The drawing under review shows one solid part. Ordinate dimensions are in mm from its lowest x, y, z. Coordinates: 2 decimals unless noted, no trailing zeros. Loops run counter-clockwise (first coordinate to the right, second up) from the corner with the lowest first, then second, coordinate; pieces in that order, holes last. Notation, with made-up numbers: (-22, -39) -> (28, -39) arc R6 ccw to (28, -35) -> close; hole circle Ø9 at (79.5, 39). An arc over 180 degrees is marked (long way). Use a Markdown table: item, result.
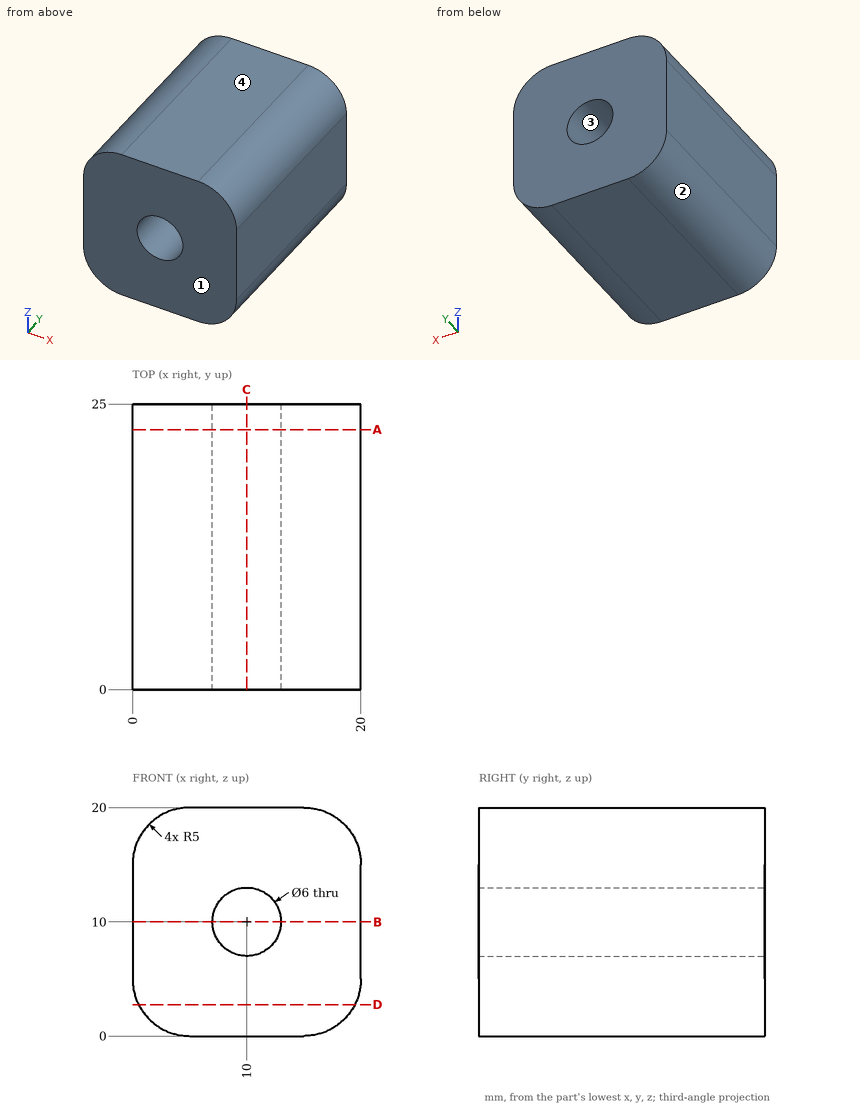
(1) Take a section at C-C on x = 10. Write out the cut boundary in (y, z), plus the area to 3 significant figures.
Found:
| item | result |
|---|---|
| outline | (0, 0) -> (25, 0) -> (25, 7) -> (0, 7) -> close; (0, 13) -> (25, 13) -> (25, 20) -> (0, 20) -> close |
| area | 350 mm^2 |
(2) Take a section at A-A on y = 22.75. Write out the cut boundary in (x, z).
Found:
| item | result |
|---|---|
| outline | (0, 5) arc R5 ccw to (5, 0) -> (15, 0) arc R5 ccw to (20, 5) -> (20, 15) arc R5 ccw to (15, 20) -> (5, 20) arc R5 ccw to (0, 15) -> close; hole circle Ø6 at (10, 10) |
(3) Mouldability with a two-part tool opening along Z and no side actions: class the marked faces 1, 2, 3 and 4 as pulls with the +Z half, pulls with the -Z half, needs draft (parallel to the pull), parting line crosses it, or undercut.
Found:
| item | result |
|---|---|
| face 1 | needs draft |
| face 2 | pulls with the -Z half |
| face 3 | undercut |
| face 4 | pulls with the +Z half |
(4) Take a section at D-D on z = 2.75. Write out the cut boundary in (x, y), plus the area to 3 significant figures.
Found:
| item | result |
|---|---|
| outline | (0.53, 0) -> (19.47, 0) -> (19.47, 25) -> (0.53, 25) -> close |
| area | 473 mm^2 |
(5) Take a section at B-B on z = 10. Write out the cut boundary in (x, y), plus the area to 3 significant figures.
Found:
| item | result |
|---|---|
| outline | (0, 0) -> (7, 0) -> (7, 25) -> (0, 25) -> close; (13, 0) -> (20, 0) -> (20, 25) -> (13, 25) -> close |
| area | 350 mm^2 |
(6) For line 1 along X through (y, z) = (12.75, 10); line 2 along X through (y, z) = (19, 11), list the stretches that pass through material, from the lowest coordinate up.
Found:
| item | result |
|---|---|
| line 1 | x = 0 to 7, 13 to 20 |
| line 2 | x = 0 to 7.17, 12.83 to 20 |
